Source: CAD feature listing. Evaluate the final solid. Frame: model axes, mm. Face numbers are marked on the shaded views. A direction names the side the tool comes from. Coordinates: 2 decimals unless noted, no trailing zeros. Order: outer loops, then holes, each group sorted by start corner. A loop starts at its lowest first (then second) coordinate and runs counter-clockwise, first axis right, second up.
Item 1: Contact query for flat-ended pins moving along their axis: P1, Ø1.2, axis at x = 4, y = 6.93, coming from the -Z side; P2, Ø8, axis at y = 5.5, z = 8.5, coming from the -X side; P3, Ø3, axis at x = 6.93, y = 4, coming from the +Z side. Output: stop coordinate, or through.
Item 2: Mould query, pull axis Y, two halves, no side actions, for the marked faces 1, 2 and 3. Classes: released by +Y, released by -Y, zero draft, split by the parting line, or undercut.
Item 3: Reachability of the marked faces 4 and 5 from +Z, -Z, +X, -X, +Y, -Y: full face, straight path, thin tool, end or side. Return the list, or none.
Item 4: Ray query, line 1 (Y direction, x = 0, z = 3.7); line 2 (Y direction, x = 4, z = 1.95); line 3 (Y direction, x = 4, z = -0.9). Return the intervals inside material, ascending.
Item 5: Section B-B on z = 6.5. Return the cut outline in (x, y).
Item 6: Section A-A on z = -2.5. Return the cut outline in (x, y).
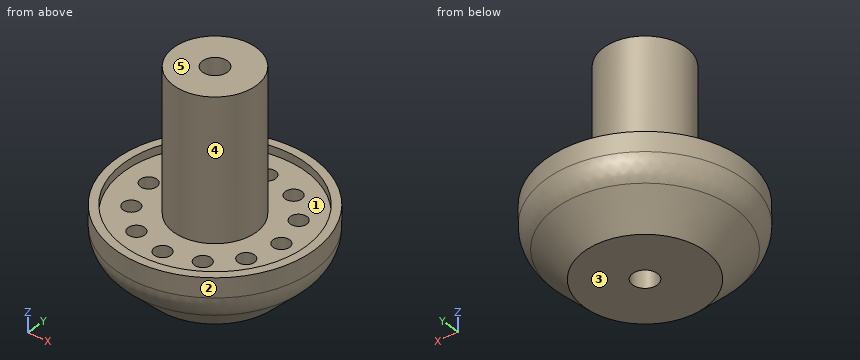
from build123d import *

# Parameters (mm, degrees)
SKETCH001_R        = 1.5
POCKET_DEPTH       = 24.646751
SKETCH002_R        = 1
POCKET001_DEPTH    = 5
POLARPATTERN_COUNT = 12
FILLET_R           = 4


with BuildPart() as part:
    # Sketch → Revolution (revolve)
    with BuildSketch(Plane.XZ):
        Polygon((0, -4.645751), (7.354249, -4.645751), (12, 0), (12, 4), (11, 4), (11, 3), (5, 3), (5, 20), (0, 20), align=None)
    revolve(axis=Axis((0, 0, 0), (0, 0, 1)))

    # Sketch001 (on Face8 of Revolution) → Pocket (cut, through all)
    with BuildSketch(Plane(origin=(0, 0, 20), x_dir=(-1, 0, 0), z_dir=(0, 0, 1))):
        Circle(SKETCH001_R)
    extrude(amount=-POCKET_DEPTH, mode=Mode.SUBTRACT)

    # Sketch002 (on Face9 of Pocket) → Pocket001 (cut)
    with BuildSketch(Plane(origin=(0, 0, 3), x_dir=(-1, 0, 0), z_dir=(0, 0, 1))):
        with Locations((-8, 0)):
            Circle(SKETCH002_R)
    pocket001 = extrude(amount=-POCKET001_DEPTH, mode=Mode.SUBTRACT)

    # PolarPattern: Pocket001 ×12 about axis
    polarpattern_axis = Axis((0, 0, 3), (0, 0, 1))
    for i in range(1, POLARPATTERN_COUNT):
        add(pocket001.rotate(polarpattern_axis, i * 360 / POLARPATTERN_COUNT), mode=Mode.SUBTRACT)

    # Fillet
    fillet_edges = [part.edges().sort_by_distance(p)[0] for p in [
        (-12, 0, 0),
    ]]
    fillet(fillet_edges, radius=FILLET_R)


solid = part.part
Answer list:
1. P1: stops at z = -4.6
1. P2: stops at x = -4.77
1. P3: stops at z = 3
2. face 1: undercut
2. face 2: split by the parting line
2. face 3: zero draft
3. face 4: +Z
3. face 5: +Z, +X, -X, +Y, -Y
4. line 1: y = -12 to -11, -5 to -1.5, 1.5 to 5, 11 to 12
4. line 2: y = -11.31 to -7.93, -5.93 to 5.93, 7.93 to 11.31
4. line 3: y = -10.33 to -7.93, -5.93 to 5.93, 7.93 to 10.33
5. outline: circle Ø10 at (0, 0); hole circle Ø3 at (0, 0)
6. outline: circle Ø19 at (0, 0); hole circle Ø3 at (0, 0)
